Autodesk Inventor part; units mm, degrees
ref_plane "YZ Plane" through (0, 0, 0) normal (1, 0, 0) x (0, 1, 0)
ref_plane "XZ Plane" through (0, 0, 0) normal (0, 1, 0) x (-1, 0, 0)
ref_plane "XY Plane" through (0, 0, 0) normal (0, 0, 1) x (1, 0, 0)
sketch "Sketch1" plane through (0, 0, 0) normal (0, 0, 1) x (1, 0, 0)
  circle A0 centre (0, 0) radius 7.874
  dimension "d0" = 15.748
extrude "Extrusion1" add sketch "Sketch1" along normal blind 67.31
ref_plane "Work Plane1" through (0, 0, 71.12) normal (0, 0, 1) x (1, 0, 0)
sketch "Sketch3" plane through (0, 0, 71.12) normal (0, 0, 1) x (1, 0, 0)
  circle A0 centre (0, 0) radius 3.81
  dimension "d4" = 7.62
loft "Loft1" add profiles "Sketch3" section 1 edges at (-7.874, 0, 67.31)
sketch "Sketch4" plane through (0, 0, 71.12) normal (0, 0, 1) x (1, 0, 0)
  circle A0 centre (0, 0) radius 3.81
  circle A1 centre (0, 0) radius 4.445
  dimension "d9" = 8.89
extrude "Extrusion2" add sketch "Sketch4" along normal blind 13.97 contours A0 | A1
sketch "Sketch5" plane through (0, 0, 85.09) normal (0, 0, 1) x (1, 0, 0)
  circle A0 centre (0, 0) radius 4.445
  point P0 (4.445, 0)
ref_plane "Work Plane2" through (4.445, 0, 85.09) normal (1, 0, 0) x (0, 1, 0)
sketch "Sketch6" plane through (4.445, 0, 85.09) normal (1, 0, 0) x (0, 1, 0)
  line L0 (4.445, 0) -> (-4.445, 0)
  point P0 (0, -85.09)
  point P1 (0, -4.826)
  dimension "d23" = 4.826
sketch "Sketch7" plane through (0, 0, 0) normal (0, 0, -1) x (-1, 0, 0)
  circle A0 centre (0, 0) radius 5.08
  dimension "d16" = 10.16
extrude "Extrusion4" add sketch "Sketch7" along normal blind 9.652
sketch "Sketch8" plane through (4.445, 0, 85.09) normal (1, 0, 0) x (0, 1, 0)
  line L0 (-5.08, -94.742) -> (5.08, -94.742)
  point P0 (0, -85.09)
  point P1 (0, -89.662)
  dimension "d31" = 5.08
hole "Hole1" at (4.445, 0, 80.264) direction (-1, 0, 0) diameter 5.08 end through all
hole "Hole2" at (4.445, 0, -4.572) direction (-1, 0, 0) diameter 5.08 end through all both
properties part number "MockShock"
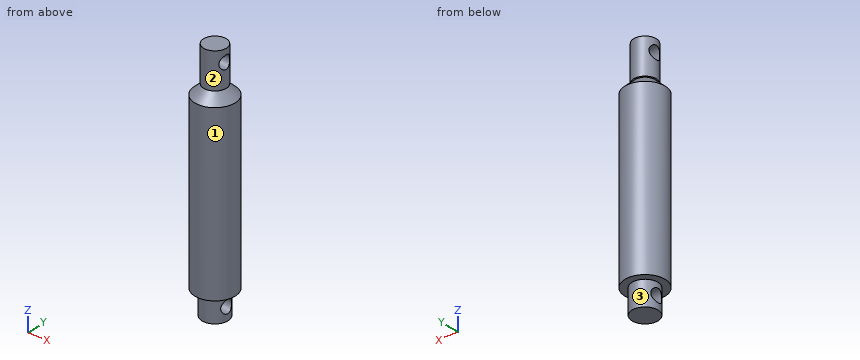
Verification items for the finished model (mm, model axes). Face numbers are marked on the shaded views. A direction names the side the tool comes from. Give positions to 0.01 mm unless a question says otherwise; leave off trailing zeros. Order: outer loops, then holes, each group sorted by start corner. A loop starts at its lowest first (then second) coordinate and runs counter-clockwise, first axis right, second up. Notation, with made-up numbers: M 59.5,45 L 86.5,45 A27 cw 86.5,78 Z; hole C 6,64.5 d2. An arc over 180 degrees is marked long. Answer in a Markdown table with one row per item. Add a question column.
Item 1: Section check C-C, the plane z = 74.5. Enter the section's corners in (x, y) (3 decimals).
Item 2: Scan lines: probe 1 along Z at (x, y) = (-0.25, 0); probe 2 along X at (y, z) = (-0.5, 18.5); probe 3 along Y at (x, z) = (6.5, 67). Record each from-to range of solid material in increasing order. Write a range as from..to.
Item 3: Section check A-A, the plane x = 0. Enter the section's corners in (y, z) (3 decimals).
Item 4: Section check D-D, the plane z = 24. Enter the section's corners in (x, y), and give its area (3 significant figures).
Item 5: Section check B-B, the plane y = 0. State how many separate pieces and enclosed holes the cut face has, and give its area (3 significant figures).
Item 6: Gauge pin test, flat ends, axial feed: pin 1 (4 mm diameter, centred on x = 2.5, z = 1.5, fed in from +Y); pin 2 (1 mm diameter, centred on y = -2, z = 49.5, fed in from -X); pin 3 (5 mm diameter, centred on x = 6.5, y = 5.5, fed in from +Z); pin 4 (4 mm diameter, centred on y = 0, z = -4.572, fed in from -X). Record the tip position at first contact, or that the pin passes through.
Item 7: Tool access check on the marked faces 1, 2 and 3. Record the directions out of +Z, -Z, +X, -X, +Y, -Y that give a thin tool (end or side, any length) a straight path to the whole face; none if there is none.
Filled sheet:
| question | item | result |
|---|---|---|
| 1 | outline | C 0,0 d8.89 |
| 2 | probe 1 | z = -9.65..-7.11, -2.03..77.72, 82.8..85.09 |
| 2 | probe 2 | x = -7.86..7.86 |
| 2 | probe 3 | y = -4.44..4.44 |
| 3 | outline | M -7.874,0 L -5.08,0 L -5.08,-9.652 L 5.08,-9.652 L 5.08,0 L 7.874,0 L 7.874,67.31 L 3.81,71.12 L 4.445,71.12 L 4.445,85.09 L -4.445,85.09 L -4.445,71.12 L -3.81,71.12 L -7.874,67.31 Z; hole C 0,-4.572 d5.08; hole C 0,80.264 d5.08 |
| 4 | outline | C 0,0 d15.75 |
| 4 | area | 195 mm^2 |
| 5 | separate pieces | 3 |
| 5 | enclosed holes | 0 |
| 5 | area | 1,230 mm^2 |
| 6 | pin 1 | stops at y = 7.86 |
| 6 | pin 2 | stops at x = -7.73 |
| 6 | pin 3 | stops at z = 69.05 |
| 6 | pin 4 | passes through |
| 7 | face 1 | +Z, -Z |
| 7 | face 2 | +Z |
| 7 | face 3 | -Z |
